Job drawing, mm, ordinate dimensions from the low corner. One solid piece. Coordinates: 2 decimals unless noted, no trailing zeros. Loops run counter-clockwise (first coordinate to the right, second up) from the corner with the lowest first, then second, coordinate; pieces in that order, holes last. Notation, with made-up numbers: (86.5, 72.5) - (104.5, 72.5) arc R19 cw to (104.5, 80.5) - close; hole circle Ø9 at (-16, 17.5). An arc over 180 degrees is marked (long way). Use a Markdown table: item, result. Add a question column.
1. Band-saw the part on B-B, the plane x = 45. Give the cut face in (y, z), plus the area to 3 significant figures.
2. Band-saw the part on C-C, the plane z = 75. Give the cut face in (x, y).
3. Drop flat-ended pins along their axis: pin 1 (6.5 mm diameter, centred on x = 75, z = 45, fed in from +Y); pin 2 (2 mm diameter, centred on y = 1.5, z = 30.5, fed in from -X). Give the stop position or say it passes through.
4. Wall check: probe 1 along Z at (x, y) = (75, 1.35); probe 2 along X at (y, z) = (2.7, 12); probe 3 along X at (y, z) = (3.65, 12.5). Give the ranges that are in metal, low to high. Write a range as [from, to].
5. Band-saw the part on D-D, the plane y = 2.45. Give the cut face in (x, z).
6. Band-saw the part on A-A, the plane z = 45. Give the cut face in (x, y), plus the area to 3 significant figures.
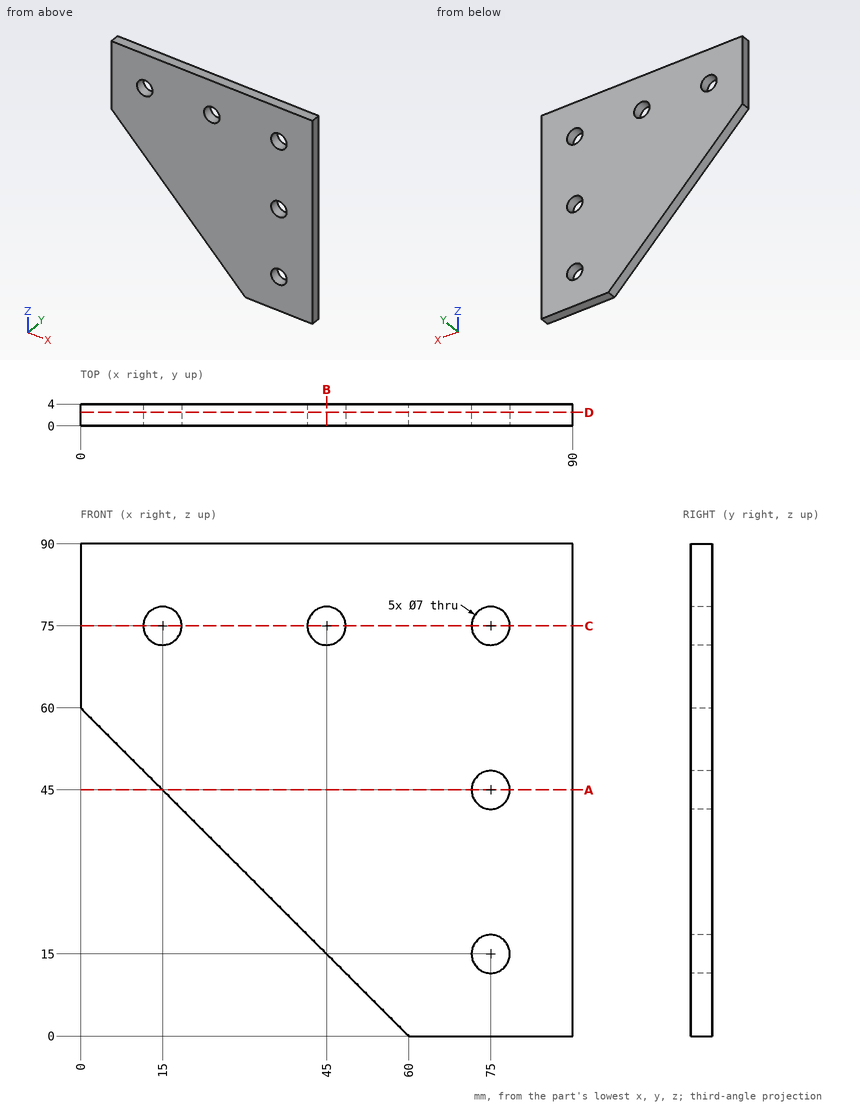
Geometry check:
| question | item | result |
|---|---|---|
| 1 | outline | (0, 15) - (4, 15) - (4, 71.5) - (0, 71.5) - close; (0, 78.5) - (4, 78.5) - (4, 90) - (0, 90) - close |
| 1 | area | 272 mm^2 |
| 2 | outline | (0, 0) - (11.5, 0) - (11.5, 4) - (0, 4) - close; (18.5, 0) - (41.5, 0) - (41.5, 4) - (18.5, 4) - close; (48.5, 0) - (71.5, 0) - (71.5, 4) - (48.5, 4) - close; (78.5, 0) - (90, 0) - (90, 4) - (78.5, 4) - close |
| 3 | pin 1 | passes through |
| 3 | pin 2 | stops at x = 28.5 |
| 4 | probe 1 | z = [0, 11.5], [18.5, 41.5], [48.5, 71.5], [78.5, 90] |
| 4 | probe 2 | x = [48, 73.2], [76.8, 90] |
| 4 | probe 3 | x = [47.5, 72.55], [77.45, 90] |
| 5 | outline | (0, 60) - (60, 0) - (90, 0) - (90, 90) - (0, 90) - close; hole circle Ø7 at (15, 75); hole circle Ø7 at (45, 75); hole circle Ø7 at (75, 15); hole circle Ø7 at (75, 45); hole circle Ø7 at (75, 75) |
| 6 | outline | (15, 0) - (71.5, 0) - (71.5, 4) - (15, 4) - close; (78.5, 0) - (90, 0) - (90, 4) - (78.5, 4) - close |
| 6 | area | 272 mm^2 |
